Input: part model. Units: mm. Frame: model coordinates. A direction names the side the tool comes from. Round coordinates to 2 decimals unless told otherwise and drop trailing zeros. Loops run counter-clockwise (first coordinate to the right, second up) from the corner with the lowest first, then second, coordinate; pieces in that order, holes last. Notation, with made-up numbers: M 14.25,85 L 43.25,85 A36 cw 43.25,121 Z; hole C 53.5,-27 d5. An arc over 180 degrees is marked long. Use one line per item in the form item = value. Start each with the question number.
Q1. Access query for faces 5 (the flat face through (0, 4, -2.3)), 6 (the flat face through (-0.3, -2, 0)), 7 (the flat face through (0, 0.6, 0)), 8 (the flat face through (0.3, -2, 0)). Directions: +Z, -Z, +X, -X, +Y, -Y. A direction counts if a zero-diameter tool reaches every point of the face in a straight line with its end or side. Return the directions, or none.
Q2. Ray query, line 1 along X through (y, z) = (1.5, -1.7); line 2 along Y through (x, z) = (-0.9, -1.45); line 3 along Y through (x, z) = (-1.45, 0.8). Return the intervals inside material, ascending.
Q3. Section query B-B, the plane z = -1.9. Output: boundary loops of the cut face in (x, y), and give its area (3 significant figures).
Q4. Section query A-A, the plane y = 1.25. Output: boundary loops of the cut face in (x, z), and give its area (3 significant figures).
Q5. First-contact query: P1, Ø2, axis at x = 1.5, z = 0, coming from the -Y side; P2, Ø1, axis at x = -1, y = -3, coming from the -Z side. Flat tips, straight axial feed; report the tip coordinate or a pass-through.
Q6. Mould query, pull axis Y, two halves, no side actions, for faces 1 (the flat face through (0, 3.4, 0)), 2 (the flat face through (0, 0, -1)), 3 (the flat face through (0, 4, 2.3)), 4 (the flat face through (1.3, 2, 0)). Classes: pulls with the +Y half, pulls with the -Y half, needs draft (parallel to the pull), parting line crosses it, or undercut.
Q7. Section query D-D, the plane z = 0.2. Output: boundary loops of the cut face in (x, y).
Q8. Section query C-C, the plane x = 0.7. Output: boundary loops of the cut face in (y, z), and give its area (3 significant figures).
```python
from build123d import *

# Parameters (mm, degrees)
SKETCH_1_W          = 3.86
SKETCH_1_H          = 4.6
EXTRUDE_1_DEPTH     = 4.6
SKETCH_2_W          = 2.6
SKETCH_2_H          = 2.8
CUT_EXTRUDE_1_DEPTH = 7.785639248
FILLET_1_R          = 0.5
FILLET_2_R          = 0.3
SKETCH_3_W          = 0.6
SKETCH_3_H          = 1
EXTRUDE_2_DEPTH     = 4.7
CHAMFER_1_SIZE      = 4.7
CHAMFER_1_SIZE_2    = 0.125
FILLET_4_R          = 0.375


with BuildPart() as part:
    # Эскиз1 → Бобышка-Вытянуть1 (new body)
    with BuildSketch(Plane(origin=(0, 0, 0), x_dir=(1, 0, 0), z_dir=(0, 1, 0))):
        Rectangle(SKETCH_1_W, SKETCH_1_H)
    extrude(amount=EXTRUDE_1_DEPTH)

    # Эскиз2 → Вырез-Вытянуть1 (cut, through all)
    with BuildSketch(Plane.XY.offset(2.3)):
        with Locations((0, 2)):
            Rectangle(SKETCH_2_W, SKETCH_2_H)
    extrude(amount=-CUT_EXTRUDE_1_DEPTH, mode=Mode.SUBTRACT)

    # Скругление1
    fillet_1_edges = [part.edges().sort_by_distance(p)[0] for p in [
        (1.93, 4.6, 0),
        (-1.93, 4.6, 0),
        (1.93, 0, 0),
        (-1.93, 0, 0),
    ]]
    fillet(fillet_1_edges, radius=FILLET_1_R)

    # Скругление2
    fillet_2_edges = [part.edges().sort_by_distance(p)[0] for p in [
        (-1.3, 0.6, 0),
        (-1.3, 3.4, 0),
        (1.3, 3.4, 0),
        (1.3, 0.6, 0),
    ]]
    fillet(fillet_2_edges, radius=FILLET_2_R)

    # Эскиз3 → Бобышка-Вытянуть2 (add)
    with BuildSketch(Plane.XZ):
        Rectangle(SKETCH_3_W, SKETCH_3_H)
    extrude(amount=EXTRUDE_2_DEPTH)

    # Фаска1
    # the kernel refuses this chamfer: 4.7, 0.125 mm, written as the material it takes off along each edge
    with BuildSketch(Plane(origin=(-12.519840253, -4.7, 0.5), x_dir=(0, 0.9999994771802269, 0.0010225650458134765), z_dir=(1, 0, 0))) as chamfer_1_piece_1_section:
        Polygon((CHAMFER_1_SIZE * 0.99999947718, -CHAMFER_1_SIZE * 0.00102256504581), (-CHAMFER_1_SIZE_2 * 0.00102256504581, -CHAMFER_1_SIZE_2 * 0.99999947718), (0, 0), align=None)
    chamfer_1_piece_1 = extrude(amount=25.039680507, mode=Mode.PRIVATE)
    chamfer_1_piece_1 = split(chamfer_1_piece_1, bisect_by=Plane(origin=(0, 0, 0.511194246), z_dir=(0, -1, 0)), keep=Keep.TOP, mode=Mode.PRIVATE)
    add(chamfer_1_piece_1, mode=Mode.SUBTRACT)
    with BuildSketch(Plane(origin=(12.519840253, -4.7, -0.5), x_dir=(0, 0.9999994771802269, -0.0010225650458134765), z_dir=(-1, 0, 0))) as chamfer_1_piece_2_section:
        Polygon((CHAMFER_1_SIZE * 0.99999947718, -CHAMFER_1_SIZE * 0.00102256504581), (-CHAMFER_1_SIZE_2 * 0.00102256504581, -CHAMFER_1_SIZE_2 * 0.99999947718), (0, 0), align=None)
    chamfer_1_piece_2 = extrude(amount=25.039680507, mode=Mode.PRIVATE)
    chamfer_1_piece_2 = split(chamfer_1_piece_2, bisect_by=Plane(origin=(0, 0, -0.511194246), z_dir=(0, -1, 0)), keep=Keep.TOP, mode=Mode.PRIVATE)
    add(chamfer_1_piece_2, mode=Mode.SUBTRACT)

    # Скругление4
    fillet_4_edges = [part.edges().sort_by_distance(p)[0] for p in [
        (0, -4.7, -0.375),
        (0, -4.7, 0.375),
    ]]
    fillet(fillet_4_edges, radius=FILLET_4_R)


solid = part.part
```
Results found:
q1.face_5 = -Z, +X, -X, +Y, -Y
q1.face_6 = +Z, -Z, -X, -Y
q1.face_7 = +Z, -Z
q1.face_8 = +Z, -Z, +X, -Y
q2.line_1 = -1.93 to -1.3, 1.3 to 1.93
q2.line_2 = 0 to 0.6, 3.4 to 4.6
q2.line_3 = 0 to 4.6
q3.outline = M -1.93,0.5 A0.5 ccw -1.43,0 L 1.43,0 A0.5 ccw 1.93,0.5 L 1.93,4.1 A0.5 ccw 1.43,4.6 L -1.43,4.6 A0.5 ccw -1.93,4.1 Z; hole M -1.3,0.9 A0.3 ccw -1,0.6 L 1,0.6 A0.3 ccw 1.3,0.9 L 1.3,3.1 A0.3 ccw 1,3.4 L -1,3.4 A0.3 ccw -1.3,3.1 Z
q3.area = 10.3 mm²
q4.outline = M -1.93,-2.3 L -1.3,-2.3 L -1.3,2.3 L -1.93,2.3 Z; M 1.3,-2.3 L 1.93,-2.3 L 1.93,2.3 L 1.3,2.3 Z
q4.area = 5.80 mm²
q5.P1 = 0
q5.P2 = through
q6.face_1 = undercut
q6.face_2 = pulls with the -Y half
q6.face_3 = needs draft
q6.face_4 = undercut
q7.outline = M -1.93,0.5 A0.5 ccw -1.43,0 L -0.3,0 L -0.3,-4.65 L 0.3,-4.65 L 0.3,0 L 1.43,0 A0.5 ccw 1.93,0.5 L 1.93,4.1 A0.5 ccw 1.43,4.6 L -1.43,4.6 A0.5 ccw -1.93,4.1 Z; hole M -1.3,0.9 A0.3 ccw -1,0.6 L 1,0.6 A0.3 ccw 1.3,0.9 L 1.3,3.1 A0.3 ccw 1,3.4 L -1,3.4 A0.3 ccw -1.3,3.1 Z
q8.outline = M 0,-2.3 L 0.6,-2.3 L 0.6,2.3 L 0,2.3 Z; M 3.4,-2.3 L 4.6,-2.3 L 4.6,2.3 L 3.4,2.3 Z
q8.area = 8.28 mm²
